Source: CAD feature listing. Evaluate the final solid. Frame: model axes, mm. Face numbers are marked on the shaded views. Round coordinates to 2 decimals unless told otherwise and drop trailing zeros. Order: outer loops, then holes, each group sorted by start corner. A loop starts at its lowest first (then second) coordinate and runs counter-clockwise, first axis right, second up. Notation, with made-up numbers: (11, 62.25) - (37, 62.25) arc R19 cw to (37, 80.25) - close; hole circle Ø8 at (10, 73.25). An arc over 180 degrees is marked (long way). Use one line per item in the form item = value. Start each with the question number.
Q1. Cut plane B-B, the plane y = 2.4. Give the number of separate pieces and of enclosed holes in the cut face, and give its area (3 significant figures).
Q2. Cut plane A-A, the plane x = 0. Return the cut outline in (y, z).
Q3. Ray query, line 1 (Z direction, x = 31.2, y = 0.2); line 2 (Z direction, x = 0, y = 2.6); line 3 (X direction, y = 1.45, z = 31.2). Return the intervals inside material, ascending. Write a range as [from, to].
Q4. Draft query along X for the marked faces 1 and 2. Return one class per face: released by +X, released by -X, zero draft, split by the parting line, or undercut.
Q5. Cut plane D-D, the plane x = -31.2. Return the cut outline in (y, z).
Q6. Cut plane C-C, the plane z = 0. Return the cut outline in (x, y), and give its area (3 significant figures).
Q7. Pin query (flat end, axial travel): pin 1 Ø8.5 at (x, z) = (-31.2, 31.2) entering from +Y; pin 2 Ø12 at (x, z) = (-23.5, -8) entering from +Y; pin 3 Ø18 at (x, z) = (0, 0) entering from -Y; pin 4 Ø4.5 at (x, z) = (9.9, -9.9) entering from +Y. Return the tip coordinate at first contact, or that it passes through.
Autodesk Inventor part; units mm, degrees
ref_plane "YZ Plane" through (0, 0, 0) normal (1, 0, 0) x (0, 1, 0)
ref_plane "XZ Plane" through (0, 0, 0) normal (0, 1, 0) x (-1, 0, 0)
ref_plane "XY Plane" through (0, 0, 0) normal (0, 0, 1) x (1, 0, 0)
sketch "Boceto1" plane through (0, 0, 0) normal (0, 1, 0) x (-1, 0, 0)
  circle A0 centre (0, 0) radius 35
  dimension "d0" = 70
extrude "Extrusión1" add sketch "Boceto1" along normal blind 3
sketch "Boceto2" plane through (0, 3, 0) normal (0, 1, 0) x (1, 0, 0)
  circle A0 centre (0, 0) radius 22.45
  circle A1 centre (0, 0) radius 32.9
  dimension "d4" = 44.9
  dimension "d5" = 65.8
extrude "Extrusión2" cut sketch "Boceto2" against normal blind 1.4
sketch "Boceto3" plane through (0, 3, 0) normal (0, 1, 0) x (1, 0, 0)
  circle A0 centre (0, 0) radius 17.5
  dimension "d8" = 35
extrude "Extrusión3" cut sketch "Boceto3" against normal through all
sketch "Boceto4" plane through (0, 3, 0) normal (0, 1, 0) x (1, 0, 0)
  circle A0 centre (0, 0) radius 17.5
  circle A1 centre (0, 0) radius 11.2
  line L0 (41.2, -41.2) -> (-41.2, -41.2)
  line L1 (-41.2, -41.2) -> (-41.2, 41.2)
  line L2 (-41.2, 41.2) -> (41.2, 41.2)
  line L3 (41.2, 41.2) -> (41.2, -41.2)
  line L4 (41.2, -41.2) -> (-41.2, 41.2) construction
  line L5 (-41.2, -41.2) -> (41.2, 41.2) construction
  circle A2 centre (0, 0) radius 35
  dimension "d11" = 22.4
  dimension "d12" = 82.4
  dimension "d13" = 82.4
extrude "Extrusión4" add sketch "Boceto4" against normal up to surface (3 mm away)
sketch "Boceto5" plane through (0, 3, 0) normal (0, 1, 0) x (1, 0, 0)
  circle A0 centre (0, 0) radius 14
  circle A1 centre (-9.8995, -9.8995) radius 1.7
  line L0 (0, 0) -> (0, -14)
  line L1 (0, 0) -> (-9.8995, -9.8995)
  circle A2 centre (-31.2, -31.2) radius 2.7
  line L2 (-41.2, 41.2) -> (-41.2, -41.2)
  line L3 (-41.2, -41.2) -> (41.2, -41.2)
  dimension "d16" = 3.4
  dimension "d17" = 28
  dimension "d18" = 45
  dimension "d21" = 10
  dimension "d22" = 10
  dimension "d23" = 5.4
extrude "Extrusión5" cut sketch "Boceto5" against normal through all contours A1 A0 | A0 L1 A1 | A1 L1 A0 | A2
sketch "Boceto6" plane through (0, 3, 0) normal (0, 1, 0) x (1, 0, 0)
  circle A0 centre (-31.2, -31.2) radius 2.7
  circle A1 centre (-31.2, -31.2) radius 4.6
  point P0 (0, 0)
  dimension "d24" = 9.2
extrude "Extrusión6" cut sketch "Boceto6" against normal blind 2
chamfer "Chaflán1" distance 1.6 angle 45 1 edges at (-11.5995, 3, 9.8995)
pattern_circular "Patrón circular1" count 4 over 360 about axis through (0, 3, 0) along (0, -1, 0) of "Extrusión5", "Extrusión6", "Chaflán1"
fillet "Empalme1" radius 5 4 edges at (-41.2, 1.5, 41.2) (41.2, 1.5, 41.2) (41.2, 1.5, -41.2) (-41.2, 1.5, -41.2)
properties part number "Motor Support Plate"
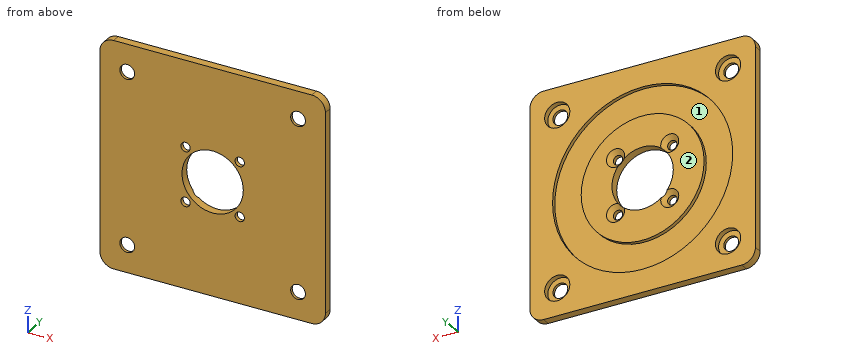
Completed:
q1.separate_pieces = 2
q1.enclosed_holes = 10
q1.area = 4,200 mm2
q2.outline = (0, -41.2) - (3, -41.2) - (3, -32.9) - (1.6, -32.9) - (1.6, -22.45) - (3, -22.45) - (3, -11.2) - (0, -11.2) - close; (0, 11.2) - (3, 11.2) - (3, 22.45) - (1.6, 22.45) - (1.6, 32.9) - (3, 32.9) - (3, 41.2) - (0, 41.2) - close
q3.line_1 = [-41.2, -33.9], [-28.5, 28.5], [33.9, 41.2]
q3.line_2 = [-41.2, -32.9], [-22.45, -11.2], [11.2, 22.45], [32.9, 41.2]
q3.line_3 = [-41.2, -35.8], [-26.6, 26.6], [35.8, 41.2]
q4.face_1 = undercut
q4.face_2 = zero draft
q5.outline = (0, -41.2) - (3, -41.2) - (3, -35.8) - (1, -35.8) - (1, -33.9) - (0, -33.9) - close; (0, -28.5) - (1, -28.5) - (1, -26.6) - (3, -26.6) - (3, -10.44) - (1.6, -10.44) - (1.6, 10.44) - (3, 10.44) - (3, 26.6) - (1, 26.6) - (1, 28.5) - (0, 28.5) - close; (0, 33.9) - (1, 33.9) - (1, 35.8) - (3, 35.8) - (3, 41.2) - (0, 41.2) - close
q6.outline = (-41.2, 0) - (-11.2, 0) - (-11.2, 3) - (-22.45, 3) - (-22.45, 1.6) - (-32.9, 1.6) - (-32.9, 3) - (-41.2, 3) - close; (11.2, 0) - (41.2, 0) - (41.2, 3) - (32.9, 3) - (32.9, 1.6) - (22.45, 1.6) - (22.45, 3) - (11.2, 3) - close
q6.area = 151 mm2
q7.pin_1 = 1
q7.pin_2 = 3
q7.pin_3 = through
q7.pin_4 = 1.95
